The model under review builds one solid part; all positions refer to its coordinate system, in mm. A direction names the side the tool comes from. Coordinates: 2 decimals unless noted, no trailing zeros. Loops run counter-clockwise (first coordinate to the right, second up) from the corner with the lowest first, then second, coordinate; pieces in that order, holes last. Notation, with made-up numbers: M -15,15 L 8,15 A24 ccw 8,33 Z; hole C -36.5,15.5 d10. An arc over 180 degrees is marked long. Use CSV: the item, a comma, the result in double quotes. Start each with the question number.
1. Tool access review of faces 5 (the cylindrical face through (26.014, -6.083, -6.633)), 6 (the flat face through (30, 0, 0)): name each direction out of +Z, -Z, +X, -X, +Y, -Y from which nothing blocks a thin tool from reaching the whole face with its end or side.
2. Add section D-D, the plane x = 11. Write out the cut boundary in (y, z), then the cut area to 3 significant figures.
3. For L1, parallel to X at y = -9, z = -4.75; L2, parallel to X at y = -8.5, z = -8.25; L3, parallel to X at y = -5.75, z = 10, list the stretches that pass through material, from the lowest coordinate up.
4. Draft analysis for pull direction X (two halves, no side actions). For faces 1 (the cylindrical face through (13.1, -11.4, -1.5)), 2 (the cylindrical face through (4.169, -3.604, 11.446)), 3 (the flat face through (0, 0, 0)), 4 (the flat face through (24.5, -4, 9)), state which applies: +X half, -X half, draft (parallel to the pull), parting line (faces both ways), or undercut.
5. Clearance check with flat-ended pins moving along their axes: P1, Ø3, axis at x = 20.5, y = 8, coming from the -Z side; P2, Ø5, axis at x = 9, y = 2.5, coming from the +Z side; P3, Ø3, axis at x = 9, z = -5.5, coming from the -Y side. State where each tip first meets the part, or that it passes through.
6. Add section C-C, the plane x = 5.75. Write out the cut boundary in (y, z).
from build123d import *


with BuildPart() as part:
    # Esquisse1 → R_volution1 (revolve)
    with BuildSketch(Plane.XY, mode=Mode.PRIVATE) as r_volution1_sk:
        with BuildLine():
            Line((0, 0), (0, 10.267949192))
            Line((0, 10.267949192), (1, 12))
            Line((1, 12), (7.25, 12))
            Line((7.25, 12), (7.25, 11.75))
            ThreePointArc((7.25, 11.75), (7.323223305, 11.573223305), (7.5, 11.5))
            Line((7.5, 11.5), (18.5, 11.5))
            ThreePointArc((18.5, 11.5), (18.676776695, 11.573223305), (18.75, 11.75))
            Line((18.75, 11.75), (18.75, 12))
            Line((18.75, 12), (24.5, 12))
            Line((24.5, 12), (24.5, 9.5))
            ThreePointArc((24.5, 9.5), (24.646446609, 9.146446609), (25, 9))
            Line((25, 9), (27, 9))
            ThreePointArc((27, 9), (27.353553391, 9.146446609), (27.5, 9.5))
            Line((27.5, 9.5), (27.5, 12))
            Line((27.5, 12), (29.744406675, 12))
            Line((29.744406675, 12), (30, 11.744406675))
            Line((30, 11.744406675), (30, 0))
            Line((30, 0), (0, 0))
        make_face()
    revolve(r_volution1_sk.sketch.rotate(Axis((-20.325204918, 0, 0), (1, 0, 0)), 90), axis=Axis((-20.325204918, 0, 0), (1, 0, 0)))


solid = part.part
Computed:
1,face 5,"none"
1,face 6,"+Z, -Z, +X, +Y, -Y"
2,outline,"C 0,0 d23"
2,area,"415 mm^2"
3,L1,"x = 0 to 24.5, 27.5 to 30"
3,L2,"x = 0.91 to 7.25, 18.75 to 24.5, 27.5 to 29.9"
3,L3,"x = 0.73 to 7.37, 18.63 to 24.5, 27.5 to 30"
4,face 1,"undercut"
4,face 2,"draft"
4,face 3,"-X half"
4,face 4,"undercut"
5,P1,"stops at z = -10.09"
5,P2,"stops at z = 11.98"
5,P3,"stops at y = -10.78"
6,outline,"C 0,0 d24"
